Part model, mm, in its own coordinate system. Face numbers are marked on the shaded views. A direction names the side the tool comes from. Coordinates: 2 decimals unless noted, no trailing zeros. Loops run counter-clockwise (first coordinate to the right, second up) from the corner with the lowest first, then second, coordinate; pieces in that order, holes last. Notation, with made-up numbers: (51.25, 32.5) -> (75.25, 32.5) arc R33 ccw to (75.25, 62.5) -> close; hole circle Ø6 at (-27, -39). An arc over 180 degrees is marked (long way). Use one line per item in the form item = value. Start each with the question number.
(1) Band-saw the part on A-A on z = 12.5. Give the cut face in (x, y).
(2) Pin check, flat tips, straight feed: P1, Ø1.5, axis at x = -1, z = 19.5, coming from the +Y side; P2, Ø1.6, axis at y = -0.5, z = 16.5, coming from the +X side; P3, Ø1.5, axis at x = -0.5, z = 21.5, coming from the -Y side. Stop position of each tip, or through.
(3) 3-axis set-ups, long thin cutter, end or side, ignore diameter. For the marked faces 1, 2, 3 and 4: which of +Z, -Z, +X, -X, +Y, -Y reach the whole face in a straight line?
(4) Drill centre lines: L1, parallel to Z at x = 6.75, y = -1.75; L2, parallel to X at y = 1.5, z = 18.5; L3, parallel to Y at x = -0.25, z = 15.75. Where is each one in solid material? Low to high. Write a range as [from, to].
(5) Band-saw the part on C-C on x = -6.5. Give the cut face in (y, z).
(6) Band-saw the part on B-B on x = -2. Give the cut face in (y, z), then the cut area to 3 significant figures.
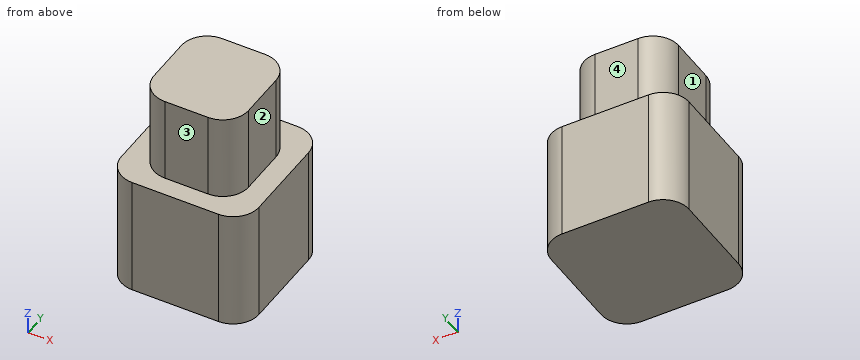
```python
from build123d import *

# Parameters (mm, degrees)
F0_W     = 16
F0_H     = 16
F1_DEPTH = 14
F2_W     = 11
F2_H     = 11.5
F3_DEPTH = 10
F4_R     = 3


with BuildPart() as f1:
    # F0 (on Top) → F1 (new body)
    with BuildSketch(Plane.XY):
        Rectangle(F0_W, F0_H)
    extrude(amount=F1_DEPTH)

    # F2 (on face) → F3 (join)
    with BuildSketch(Plane.XY.offset(14)):
        Rectangle(F2_W, F2_H)
    extrude(amount=F3_DEPTH)

    # F4
    f4_edges = [f1.edges().sort_by_distance(p)[0] for p in [
        (5.5, -5.75, 19),
        (5.5, 5.75, 19),
        (-5.5, -5.75, 19),
        (-8, -8, 7),
        (8, -8, 7),
        (8, 8, 7),
        (-8, 8, 7),
        (-5.5, 5.75, 19),
    ]]
    fillet(f4_edges, radius=F4_R)


solid = f1.part
```
A:
q1.outline = (-8, -5) arc R3 ccw to (-5, -8) -> (5, -8) arc R3 ccw to (8, -5) -> (8, 5) arc R3 ccw to (5, 8) -> (-5, 8) arc R3 ccw to (-8, 5) -> close
q2.P1 = 5.75
q2.P2 = 5.5
q2.P3 = -5.75
q3.face_1 = +Z, -X, +Y, -Y
q3.face_2 = +Z, +X, +Y, -Y
q3.face_3 = +Z, +X, -X, -Y
q3.face_4 = +Z, +X, -X, +Y
q4.L1 = [0, 14]
q4.L2 = [-5.5, 5.5]
q4.L3 = [-5.75, 5.75]
q5.outline = (-7.6, 0) -> (7.6, 0) -> (7.6, 14) -> (-7.6, 14) -> close
q6.outline = (-8, 0) -> (8, 0) -> (8, 14) -> (5.75, 14) -> (5.75, 24) -> (-5.75, 24) -> (-5.75, 14) -> (-8, 14) -> close
q6.area = 339 mm²
